from build123d import *

# Parameters (mm, degrees)
CENTER_DEPTH         = 23
CENTER_DEPTH_BACK    = 23
ANGLE_CUT_DEPTH      = 29.472794032
ANGLE_CUT_DEPTH_BACK = 29.472794032
END_DEPTH            = 25
FILLET2_R            = 1.5
SKETCH10_W           = 8.6
SKETCH10_H           = 8.6
SQUARE_HOLE_DEPTH    = 18.6
ROUND_HOLE_REACH     = 53.623
SKETCH11_R           = 3.1
FILLET2_OF_MIRROR2_R = 1.5


with BuildPart() as part:
    # Sketch1 → Center (new, two sides: drawn at the far end of the back side and taken through both)
    with BuildSketch(Plane.ZY.offset(-CENTER_DEPTH_BACK)):
        with BuildLine():
            Line((6.9, 8.4), (6.9, -8.4))
            ThreePointArc((6.9, -8.4), (0, -15.3), (-6.9, -8.4))
            Line((-6.9, -8.4), (-6.9, 8.4))
            ThreePointArc((-6.9, 8.4), (0, 15.3), (6.9, 8.4))
        make_face()
    extrude(amount=CENTER_DEPTH + CENTER_DEPTH_BACK)

    # Sketch8 → Angle Cut (cut, two sides: drawn at the far end of the back side and taken through both)
    with BuildSketch(Plane(origin=(0, 0, 0), x_dir=(1, 0, 0), z_dir=(0, 1, 0)).offset(-ANGLE_CUT_DEPTH_BACK)):
        Polygon((-32.849207695, 10), (-22.849207695, 10), (-22.150792305, -10), (-32.849207695, -10), align=None)
        Polygon((32.849207695, -10), (22.150792305, -10), (22.849207695, 10), (32.849207695, 10), align=None)
    extrude(amount=ANGLE_CUT_DEPTH + ANGLE_CUT_DEPTH_BACK, mode=Mode.SUBTRACT)

    # Sketch9 → End (add)
    with BuildSketch(Plane(origin=(22.472595565, 0, 0.78476033), x_dir=(0.03489949670249425, 0, -0.999390827019096), z_dir=(0.999390827019096, 0, 0.03489949670249425))):
        with BuildLine():
            Line((-5.114761324, -7.9), (-5.114761324, 7.9))
            ThreePointArc((-5.114761324, 7.9), (0.785238676, 13.8), (6.685238676, 7.9))
            Line((6.685238676, 7.9), (6.685238676, -7.9))
            ThreePointArc((6.685238676, -7.9), (0.785238676, -13.8), (-5.114761324, -7.9))
        make_face()
    end = extrude(amount=END_DEPTH)

    # Fillet2
    fillet2_edges = [part.edges().sort_by_distance(p)[0] for p in [
        (47.484770675, -13.8, 0.872487418),
        (47.690677706, 0, -5.023918462),
        (47.484770675, 13.8, 0.872487418),
        (47.278863645, 0, 6.768893297),
    ]]
    fillet(fillet2_edges, radius=FILLET2_R)

    # Sketch10 → Square Hole (cut)
    with BuildSketch(Plane(origin=(47.457366241, 0, 1.657247747), x_dir=(0.03489949670249425, 0, -0.999390827019096), z_dir=(0.999390827019096, 0, 0.03489949670249425))):
        with Locations((0.785238676, 0)):
            Rectangle(SKETCH10_W, SKETCH10_H)
    square_hole = extrude(amount=-SQUARE_HOLE_DEPTH, mode=Mode.SUBTRACT)

    # Sketch11 → Round Hole (cut, up to next)
    with BuildSketch(Plane(origin=(-0.178502596, 0, 5.11164555), x_dir=(0.999390827019096, 0, 0.03489949670249425), z_dir=(-0.03489949670249425, 0, 0.999390827019096)), mode=Mode.PRIVATE) as round_hole_sk1:
        with Locations((35.986293608, 0)):
            Circle(SKETCH11_R)
    round_hole_tool1 = extrude(round_hole_sk1.sketch, amount=-ROUND_HOLE_REACH, mode=Mode.PRIVATE) & part.part
    round_hole = round_hole_tool1.solids().sort_by_distance((35.785869, 0, 6.367549))[0]
    add(round_hole, mode=Mode.SUBTRACT)

    # Mirror2: End, Square Hole, Round Hole across plane
    add(end.mirror(Plane(origin=(0, 0, 0), x_dir=(0, 0, 1), z_dir=(1, 0, 0))))
    add(square_hole.mirror(Plane(origin=(0, 0, 0), x_dir=(0, 0, 1), z_dir=(1, 0, 0))), mode=Mode.SUBTRACT)
    add(round_hole.mirror(Plane(origin=(0, 0, 0), x_dir=(0, 0, 1), z_dir=(1, 0, 0))), mode=Mode.SUBTRACT)

    # Fillet2 of Mirror2
    fillet2_of_mirror2_edges = [part.edges().sort_by_distance(p)[0] for p in [
        (-47.484770675, -13.8, 0.872487418),
        (-47.690677706, 0, -5.023918462),
        (-47.484770675, 13.8, 0.872487418),
        (-47.278863645, 0, 6.768893297),
    ]]
    fillet(fillet2_of_mirror2_edges, radius=FILLET2_OF_MIRROR2_R)


solid = part.part
The listing builds one solid part. Answer for the finished solid, in the listing's coordinates (mm). Round coordinates to 2 decimals unless told otherwise and drop trailing zeros. Loops run counter-clockwise (first coordinate to the right, second up) from the corner with the lowest first, then second, coordinate; pieces in that order, holes last. Notation, with made-up numbers: M 76.5,-6 L 91.5,-6 A16 cw 91.5,10 Z; hole C 13,58.5 d3. An arc over 180 degrees is marked long. Write each question's results on one line, items separated by ' | '. Start each with the question number.
1) Each of these flat-tipped pins is pushed along its axis until it touches: pin 1 (5 mm diameter, centred on x = 35.5, y = -3, fed in from +Z); pin 2 (4.5 mm diameter, centred on x = 41.5, z = 1, fed in from +Y); pin 3 (4.5 mm diameter, centred on x = 38, z = 0, fed in from -Y). Where does it stop, or does it pass through?
2) Find section A-A on x = 13. Write down the section's boundary in (y, z), plus the area to 3 significant figures.
3) Determine the mould class of faces 1 (the cylindrical face through (34.1, 13.8, 0.5)), 2 (the cylindrical face through (-46.84, 0.11, 6.33)), 3 (the flat face through (38, 4.3, 1)) for opening direction Y: pulls with the +Y half, pulls with the -Y half, needs draft (parallel to the pull), parting line crosses it, or undercut.
4) Straight lines are drawn through the part: probe 1 along Y at (x, z) = (40, 3); probe 2 along Y at (x, z) = (-44, 3.25); probe 3 along Z at (x, y) = (-19.5, 12). For each, find the intervals that lie inside material, in ascending order.
Final values:
1) pin 1: z = 6.44 | pin 2: y = 13.8 | pin 3: y = -13.8
2) outline: M -8.4,-6.9 L 8.4,-6.9 A6.9 ccw 8.4,6.9 L -8.4,6.9 A6.9 ccw Z | area: 381 mm²
3) face 1: pulls with the +Y half | face 2: needs draft | face 3: undercut
4) probe 1: -13.3 to -4.3, 4.3 to 13.3 | probe 2: -13.25 to -4.3, 4.3 to 13.25 | probe 3: -5.89 to 5.89
